Design review of the part built by this model. Coordinates are the model's own, in mm. A direction names the side the tool comes from. Round coordinates to 2 decimals unless told otherwise and drop trailing zeros. Write each loop counter-clockwise with the first axis right and the second up, starting at its lowest first coordinate (ties: lowest second). Pieces come first, ordered by that corner, then holes. Notation, with made-up numbers: (82, -38) - (131, -38) arc R14 ccw to (131, -23) - close; hole circle Ø10 at (-35, -0.75). An arc over 180 degrees is marked (long way). Use one line per item in the form item = value.
```python
from build123d import *

# Parameters (mm, degrees)
SKIZZE2_W                                    = 40
SKIZZE2_H                                    = 15
AUFSATZ_LINEAR_AUSTRAGEN1_DEPTH              = 90
SKIZZE3_R                                    = 5
SCHNITT_LINEAR_AUSTRAGEN1_DEPTH              = 80
SKIZZE4_R                                    = 4
SCHNITT_LINEAR_AUSTRAGEN2_DEPTH              = 5
SKIZZE5_R                                    = 1.1
SCHNITT_LINEAR_AUSTRAGEN3_DEPTH              = 91.691785736
STIRNSENKUNG_F_R_M2_FLACHKOPFSCHRAUB_2_COUNT = 2
STIRNSENKUNG_F_R_M2_FLACHKOPFSCHRAUB_2_PITCH = 50
STIRNSENKUNG_F_R_M2_FLACHKOPFSCHRAUB_3_COUNT = 2
STIRNSENKUNG_F_R_M2_FLACHKOPFSCHRAUB_3_PITCH = 57.306195128
STIRNSENKUNG_F_R_M2_FLACHKOPFSCHRAUB_4_COUNT = 2
STIRNSENKUNG_F_R_M2_FLACHKOPFSCHRAUB_4_PITCH = 28
SCHNITT_LINEAR_AUSTRAGEN6_DEPTH              = 100.624294226
SCHNITT_LINEAR_AUSTRAGEN6_DEPTH_BACK         = 100.624294226
SCHNITT_LINEAR_AUSTRAGEN7_DEPTH              = 100.624294371
SCHNITT_LINEAR_AUSTRAGEN7_DEPTH_BACK         = 100.624294371


with BuildPart() as part:
    # Skizze2 → Aufsatz-Linear austragen1 (new body)
    with BuildSketch(Plane(origin=(0, 0, 0), x_dir=(1, 0, 0), z_dir=(0, 1, 0))):
        with Locations((20, 7.5)):
            Rectangle(SKIZZE2_W, SKIZZE2_H)
    extrude(amount=AUFSATZ_LINEAR_AUSTRAGEN1_DEPTH)

    # Skizze3 → Schnitt-Linear austragen1 (cut)
    with BuildSketch(Plane(origin=(0, 90, 0), x_dir=(1, 0, 0), z_dir=(0, 1, 0))):
        with Locations((20, 0)):
            Circle(SKIZZE3_R)
    extrude(amount=-SCHNITT_LINEAR_AUSTRAGEN1_DEPTH, mode=Mode.SUBTRACT)

    # Skizze4 → Schnitt-Linear austragen2 (cut)
    with BuildSketch(Plane.XZ):
        with Locations((20, 0)):
            Circle(SKIZZE4_R)
    extrude(amount=-SCHNITT_LINEAR_AUSTRAGEN2_DEPTH, mode=Mode.SUBTRACT)

    # Skizze5 → Schnitt-Linear austragen3 (cut, through all)
    with BuildSketch(Plane(origin=(0, 10, 0), x_dir=(1, 0, 0), z_dir=(0, 1, 0))):
        with Locations((20, 0)):
            Circle(SKIZZE5_R)
    extrude(amount=-SCHNITT_LINEAR_AUSTRAGEN3_DEPTH, mode=Mode.SUBTRACT)

    # Skizze8 → Stirnsenkung für M2 Flachkopfschraube mit Schlitz1 (revolve, cut)
    with BuildSketch(Plane(origin=(6, 70, -15), x_dir=(0, 1, 0), z_dir=(1, 0, 0))):
        Polygon((0, 0), (0, 15), (1.1, 15), (1.1, 12.6), (2.5, 12.6), (2.5, 1), (3.5, 0), align=None)
    stirnsenkung_f_r_m2_flachkopfschraube_mi = revolve(axis=Axis((6, 70, -21.35), (0, 0, 1)), mode=Mode.SUBTRACT)

    # Stirnsenkung f_r M2 Flachkopfschraub 2: Stirnsenkung für M2 Flachkopfschraube mit Schlitz1 ×2
    with Locations(*[(0, -i * STIRNSENKUNG_F_R_M2_FLACHKOPFSCHRAUB_2_PITCH, 0) for i in range(1, STIRNSENKUNG_F_R_M2_FLACHKOPFSCHRAUB_2_COUNT)]):
        add(stirnsenkung_f_r_m2_flachkopfschraube_mi, mode=Mode.SUBTRACT)

    # Stirnsenkung f_r M2 Flachkopfschraub 3: Stirnsenkung für M2 Flachkopfschraube mit Schlitz1 ×2
    with Locations(*[Vector(0.48860336893184336, -0.87250601594972, 0) * (i * STIRNSENKUNG_F_R_M2_FLACHKOPFSCHRAUB_3_PITCH) for i in range(1, STIRNSENKUNG_F_R_M2_FLACHKOPFSCHRAUB_3_COUNT)]):
        add(stirnsenkung_f_r_m2_flachkopfschraube_mi, mode=Mode.SUBTRACT)

    # Stirnsenkung f_r M2 Flachkopfschraub 4: Stirnsenkung für M2 Flachkopfschraube mit Schlitz1 ×2
    with Locations(*[(i * STIRNSENKUNG_F_R_M2_FLACHKOPFSCHRAUB_4_PITCH, 0, 0) for i in range(1, STIRNSENKUNG_F_R_M2_FLACHKOPFSCHRAUB_4_COUNT)]):
        add(stirnsenkung_f_r_m2_flachkopfschraube_mi, mode=Mode.SUBTRACT)

    # Skizze11 → Schnitt-Linear austragen6 (cut, two sides: drawn at the far end of the back side and taken through both)
    with BuildSketch(Plane(origin=(0, 90, 0), x_dir=(1, 0, 0), z_dir=(0, 1, 0)).offset(-SCHNITT_LINEAR_AUSTRAGEN6_DEPTH_BACK)):
        with BuildLine():
            Line((130.666560763, 23.133312153), (40, 5))
            ThreePointArc((40, 5), (30.428932188, 6.893398282), (25, 15))
            Line((25, 15), (6.866687847, 105.666560763))
            Line((6.866687847, 105.666560763), (109.444191755, 259.532816625))
            Line((109.444191755, 259.532816625), (233.244064671, 176.999568015))
            Line((233.244064671, 176.999568015), (130.666560763, 23.133312153))
        make_face()
    extrude(amount=SCHNITT_LINEAR_AUSTRAGEN6_DEPTH + SCHNITT_LINEAR_AUSTRAGEN6_DEPTH_BACK, mode=Mode.SUBTRACT)

    # Skizze14 → Schnitt-Linear austragen7 (cut, two sides: drawn at the far end of the back side and taken through both)
    with BuildSketch(Plane(origin=(0, 90, 0), x_dir=(1, 0, 0), z_dir=(0, 1, 0)).offset(-SCHNITT_LINEAR_AUSTRAGEN7_DEPTH_BACK)):
        with BuildLine():
            Line((33.1333122, 105.666561001), (15, 15))
            ThreePointArc((15, 15), (9.571067812, 6.893398282), (0, 5))
            Line((0, 5), (-90.666561001, 23.1333122))
            Line((-90.666561001, 23.1333122), (-193.244065178, 176.999568466))
            Line((-193.244065178, 176.999568466), (-69.444191977, 259.532817267))
            Line((-69.444191977, 259.532817267), (33.1333122, 105.666561001))
        make_face()
    extrude(amount=SCHNITT_LINEAR_AUSTRAGEN7_DEPTH + SCHNITT_LINEAR_AUSTRAGEN7_DEPTH_BACK, mode=Mode.SUBTRACT)


solid = part.part
```
Q1. We need section C-C on y = 39. Write out the cut boundary in (x, z), then the cut area to 3 significant figures.
Calculated:
outline = (0, -5) arc R12.75 cw to (15, -15) - (25, -15) arc R12.75 cw to (40, -5) - (40, 0) - (25, 0) arc R5 cw to (15, 0) - (0, 0) - close
area = 318 mm2
Q2. Machinability: for faces 4 (the cylindrical face through (31.52, 69.67, -3.93)), 5 (the flat face through (20, 10, -3)), 6 (the flat face through (20, 5, -2)), which of the approach directions +Z, -Z, +X, -X, +Y, -Y give a long, thin tool a straight path to every point of the face, cutting with its end or side? Answer none if there is none.
Calculated:
face_4 = -Z
face_5 = +Z, +Y
face_6 = +Z, -Y
Q3. We need section B-B on x = 6. Write out the cut boundary in (y, z).
Calculated:
outline = (0, -5.24) - (17.5, -5.24) - (17.5, -2.4) - (18.9, -2.4) - (18.9, 0) - (0, 0) - close; (21.1, -2.4) - (22.5, -2.4) - (22.5, -5.24) - (67.5, -5.24) - (67.5, -2.4) - (68.9, -2.4) - (68.9, 0) - (21.1, 0) - close; (71.1, -2.4) - (72.5, -2.4) - (72.5, -5.24) - (90, -5.24) - (90, 0) - (71.1, 0) - close
Q4. For P1, Ø4, axis at x = 34, y = 20, coming from the +Z side; P2, Ø4, axis at x = 6, y = 21, coming from the -Z side; P3, Ø6, axis at y = 44, z = -11.5, coming from the -X side; P4, Ø2.5, axis at x = 34, y = 70, coming from the -Z side, all flat-tipped, find the tip position at first contact; note any pin that passes through.
Calculated:
P1 = 0
P2 = -5.95
P3 = 11.53
P4 = -2.4
Q5. Draft analysis for pull direction Y (two halves, no side actions). For faces 1 (the flat face through (35, 19, -2.4)), 2 (the cylindrical face through (20, 51, -5)), 3 (the flat face through (20, 0, -6)), state which applies: released by +Y, released by -Y, zero draft, split by the parting line, or undercut.
Calculated:
face_1 = undercut
face_2 = zero draft
face_3 = released by -Y
Q6. To check wall thickness, follow line 1 along Y through (x, z) = (6, -1); line 2 along Y through (x, z) = (6, -4.5); line 3 along X through (y, z) = (20, -1.1). State the ranges of each line that lie inside material, in increasing order. Write a range as from..to.
Calculated:
line_1 = 0..18.9, 21.1..68.9, 71.1..90
line_2 = 0..17.5, 22.5..67.5, 72.5..90
line_3 = 0..4.9, 7.1..15.12, 24.88..32.9, 35.1..40
Q7. We need section D-D on x = 20. Write out the cut boundary in (y, z).
Calculated:
outline = (0, -15) - (90, -15) - (90, -5) - (10, -5) - (10, -1.1) - (5, -1.1) - (5, -4) - (0, -4) - close
Q8. We need section A-A on y = 70. Write out the cut boundary in (x, z).
Calculated:
outline = (0, -5) arc R12.75 cw to (3.5, -4.79) - (3.5, -2.4) - (4.9, -2.4) - (4.9, 0) - (0, 0) - close; (7.1, -2.4) - (8.5, -2.4) - (8.5, -6.25) arc R12.75 cw to (15, -15) - (25, -15) arc R12.75 cw to (31.5, -6.25) - (31.5, -2.4) - (32.9, -2.4) - (32.9, 0) - (25, 0) arc R5 cw to (15, 0) - (7.1, 0) - close; (35.1, -2.4) - (36.5, -2.4) - (36.5, -4.79) arc R12.75 cw to (40, -5) - (40, 0) - (35.1, 0) - close
